Source: CAD feature listing. Evaluate the final solid. Frame: model axes, mm. Face numbers are marked on the shaded views. A direction names the side the tool comes from. Round coordinates to 2 decimals unless told otherwise and drop trailing zeros. Loops run counter-clockwise (first coordinate to the right, second up) from the corner with the lowest first, then second, coordinate; pieces in that order, holes last. Notation, with made-up numbers: (61, 15.25) -> (75, 15.25) arc R29 cw to (75, 53.25) -> close; hole circle Ø2 at (77.25, -2). An arc over 180 degrees is marked (long way). Return JSON: item names as keys, results as strings. Group by question number.
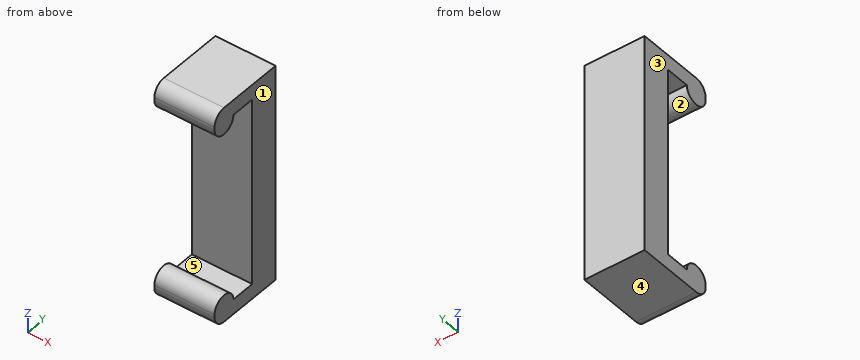
```python
from build123d import *

# Parameters (mm, degrees)
PAD_DEPTH = 4
FILLET_R  = 0.8


with BuildPart() as part:
    # Sketch → Pad (new body)
    with BuildSketch(Plane.YZ):
        with BuildLine():
            Line((1.6, 6.25), (0, 6.25))
            ThreePointArc((-1.6, 6.25), (-0.8, 5.45), (0, 6.25))
            Line((-1.6, 6.25), (-1.6, 7.25))
            Line((-1.6, 7.25), (3.6, 7.25))
            Line((3.6, 7.25), (3.6, -7.25))
            Line((3.6, -7.25), (-1.6, -7.25))
            Line((-1.6, -7.25), (-1.6, -6.25))
            ThreePointArc((0, -6.25), (-0.8, -5.45), (-1.6, -6.25))
            Line((0, -6.25), (1.6, -6.25))
            Line((1.6, -6.25), (1.6, 6.25))
        make_face()
    extrude(amount=PAD_DEPTH)

    # Fillet
    fillet_edges = [part.edges().sort_by_distance(p)[0] for p in [
        (2, -1.6, 7.25),
        (2, -1.6, -7.25),
    ]]
    fillet(fillet_edges, radius=FILLET_R)


solid = part.part
```
(1) Set-up query: the marked faces 1 and 2. Return all of +Z, -Z, +X, -X, +Y, -Y with unobstructed straight access to the full face (end or side cutting, diameter ignored); none if empty.
(2) Cut plane B-B (z = 5.75). Return loops of the section in (x, y), and give its area (3 significant figures).
(3) Cut plane C-C (x = 1.8). Return loops of the section in (y, z).
(4) Ray query, line 1 (Z direction, x = 2.9, y = 1.3); line 2 (Y direction, x = 0.35, z = -5.25); line 3 (Z direction, x = 3.8, y = -0.65). Return the intervals inside material, ascending.
(5) Cut plane A-A (y = 1.25). Return loops of the section in (x, z).
(6) Cut plane D-D (z = -4.75). Return loops of the section in (x, y), and give its area (3 significant figures).
(7) Mould query, pull axis Z, two halves, no side actions, for the marked faces 3, 4 and 5. Classes: released by +Z, released by -Z, zero draft, split by the parting line, or undercut.
Answers follow:
{
 "1": {"face 1": "+Z, -Z, +X, +Y, -Y", "face 2": "+X, -X"},
 "2": {"outline": "(0, -1.42) -> (4, -1.42) -> (4, -0.18) -> (0, -0.18) -> close; (0, 1.6) -> (4, 1.6) -> (4, 3.6) -> (0, 3.6) -> close", "area": "13.0 mm^2"},
 "3": {"outline": "(-1.6, -6.45) arc R0.8 ccw to (-0.8, -7.25) -> (3.6, -7.25) -> (3.6, 7.25) -> (-0.8, 7.25) arc R0.8 ccw to (-1.6, 6.45) -> (-1.6, 6.25) arc R0.8 ccw to (0, 6.25) -> (1.6, 6.25) -> (1.6, -6.25) -> (0, -6.25) arc R0.8 ccw to (-1.6, -6.25) -> close"},
 "4": {"line 1": "-7.25 to -6.25, 6.25 to 7.25", "line 2": "1.6 to 3.6", "line 3": "-7.25 to -5.46, 5.46 to 7.25"},
 "5": {"outline": "(0, -7.25) -> (4, -7.25) -> (4, -6.25) -> (0, -6.25) -> close; (0, 6.25) -> (4, 6.25) -> (4, 7.25) -> (0, 7.25) -> close"},
 "6": {"outline": "(0, 1.6) -> (4, 1.6) -> (4, 3.6) -> (0, 3.6) -> close", "area": "8.00 mm^2"},
 "7": {"face 3": "zero draft", "face 4": "released by -Z", "face 5": "undercut"}
}
